Autodesk Inventor part; units mm, degrees
ref_plane "YZ Plane" through (0, 0, 0) normal (1, 0, 0) x (0, 1, 0)
ref_plane "XZ Plane" through (0, 0, 0) normal (0, 1, 0) x (-1, 0, 0)
ref_plane "XY Plane" through (0, 0, 0) normal (0, 0, 1) x (1, 0, 0)
sketch "Sketch1" plane through (0, 0, 0) normal (1, 0, 0) x (0, 1, 0)
  line L0 (0, 150) -> (0, -150) construction
  line L1 (-23.875, 150) -> (-23.875, -150)
  line L2 (23.875, -150) -> (23.875, 150)
  arc A0 (23.875, 150) -> (-23.875, 150) centre (0, 150) ccw
  arc A1 (-23.875, -150) -> (23.875, -150) centre (0, -150) ccw
  line L3 (0, 0) -> (300, 0) construction
  line L4 (25.375, 150) -> (25.375, -150)
  arc A2 (-25.375, -150) -> (25.375, -150) centre (0, -150) ccw
  line L5 (-25.375, -150) -> (-25.375, 150)
  arc A3 (25.375, 150) -> (-25.375, 150) centre (0, 150) ccw
  line L6 (21.775, 150) -> (21.775, -150)
  arc A4 (-21.775, -150) -> (21.775, -150) centre (0, -150) ccw
  line L7 (-21.775, -150) -> (-21.775, 150)
  arc A5 (21.775, 150) -> (-21.775, 150) centre (0, 150) ccw
  dimension "d0" = 150
  dimension "d1" = 90
  dimension "d2" = 47.75
  dimension "d3" = 1.5
  dimension "d4" = 2.1
extrude "Extrusion1" add sketch "Sketch1" along normal blind 15 contours A0 L2 A1 L1 | L4 A2 L5 A3
properties part number "Belt 750" material "Rubber"
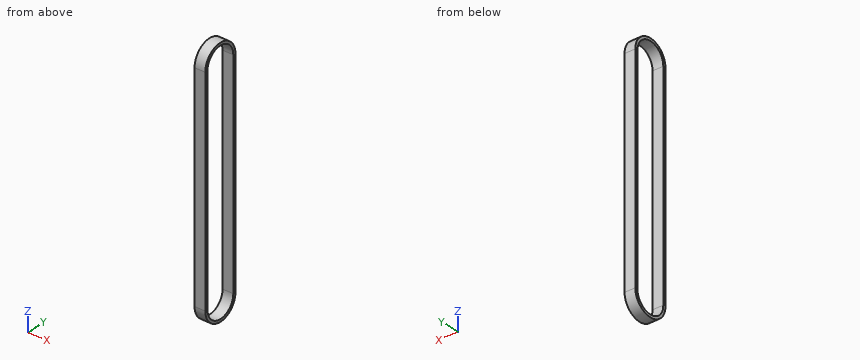
Input: part model. Units: mm. Frame: model coordinates. Give positions to 0.01 mm unless a question says otherwise; leave off trailing zeros. Order: outer loops, then holes, each group sorted by start corner. A loop starts at its lowest first (then second) coordinate and runs counter-clockwise, first axis right, second up. Notation, with made-up numbers: M 16,-30.5 L 32,-30.5 A21 cw 32,4.5 Z; hole C 41,-28 d10. An arc over 180 degrees is marked long. Answer as a JSON object with one key per item and string values.
1. Cut plane A-A, the plane z = 80.5. Output: boundary loops of the cut face in (x, y) (3 decimals).
Result sheet:
{"outline": "M 0,-25.375 L 15,-25.375 L 15,-21.775 L 0,-21.775 Z; M 0,21.775 L 15,21.775 L 15,25.375 L 0,25.375 Z"}
2. Cut plane B-B, the plane y = 0. Output: boundary loops of the cut face in (x, z) (3 decimals).
Result sheet:
{"outline": "M 0,-175.375 L 15,-175.375 L 15,-171.775 L 0,-171.775 Z; M 0,171.775 L 15,171.775 L 15,175.375 L 0,175.375 Z"}
3. Ray query, line 1 (Y direction, x = 5.75, z = -45) (3 decimals); line 2 (Z direction, x = 4.75, y = 0) (3 decimals); line 3 (Z direction, x = 8.75, y = 15.5). Return the intervals inside material, ascending. Write a range as [from, to].
Result sheet:
{"line 1": "[-25.375, -21.775], [21.775, 25.375]", "line 2": "[-175.375, -171.775], [171.775, 175.375]", "line 3": "[-170.09, -165.29], [165.29, 170.09]"}
4. Cut plane C-C, the plane x = 4.25. Output: boundary loops of the cut face in (y, z) (3 decimals), and give its area (3 significant figures).
Result sheet:
{"outline": "M -25.375,-150 A25.375 ccw 25.375,-150 L 25.375,150 A25.375 ccw -25.375,150 Z; hole M -21.775,-150 A21.775 ccw 21.775,-150 L 21.775,150 A21.775 ccw -21.775,150 Z", "area": "2,690 mm²"}
5. First-contact query: P1, Ø6, axis at x = 4.5, y = 18.5, coming from the +Z side. Flat tip, straight axial feed; report the tip coordinate or a pass-through.
Result sheet:
{"P1": "z = 170.09"}
